Geometry: see drawing. Coordinates: mm, zero at the bounding-box minimum. Give positions to 0.01 mm unless a question says otherwise; leave off trailing zeros. Order: outer loops, then holes, each group sorted by start corner. A loop starts at its lowest first (then second) coordinate and runs counter-clockwise, first axis right, second up. Notation, with made-up numbers: (43, 20) - (82, 20) arc R10 cw to (82, 29) - close; hole circle Ø8 at (-12.75, 58). An arc over 180 degrees is marked (long way). One line per question, with ' | ' between items. Start each with the question number.
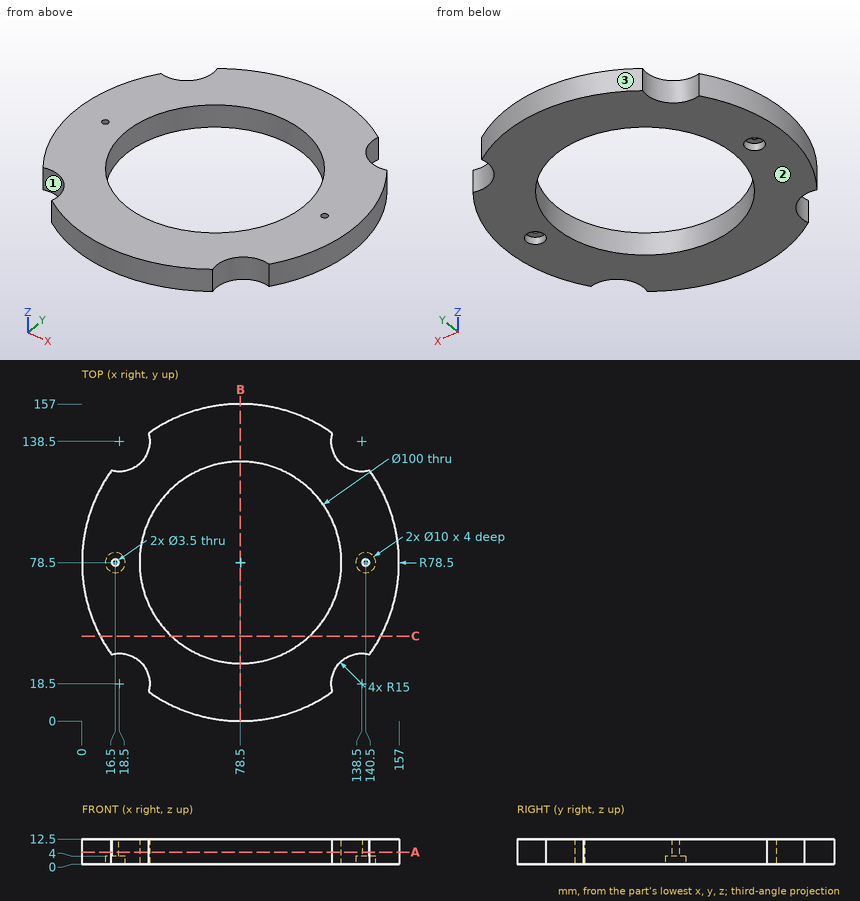
(1) Cut plane A-A, the plane z = 6. Return the cut outline in (x, y), plus the area to 3 significant figures.
(2) Pull-direction query (X, two-part tool) for the marked faces 1, 2 and 3; classes: +X half, -X half, draft (parallel to the pull), parting line (faces both ways), or undercut.
(3) Cut plane B-B, the plane x = 78.5. Return the cut outline in (y, z).
(4) Contact query for flat-ended pins moving along their axis: P1, Ø8, axis at x = 141, y = 78.5, coming from the -Z side; P2, Ø5, axis at y = 43.5, z = 5, coming from the +X side; P3, Ø2, axis at x = 16.5, y = 78.5, coming from the -Z side; P4, Ø1.5, axis at y = 22, z = 9.5, coming from the -X side. Output: stop coordinate, or through.
(5) Cut plane C-C, the plane y = 42. Return the cut outline in (x, z).
(6) Material intervals for line 1 along Y through (x, z) = (78.5, 9.25); line 2 along X through (y, z) = (106, 9.5); line 3 along Y through (x, z) = (113.5, 8.5), sorted ascending. Write a range as from..to.
Results are:
1) outline: (14.55, 32.97) arc R15 cw to (32.97, 14.55) arc R78.5 ccw to (124.03, 14.55) arc R15 cw to (142.45, 32.97) arc R78.5 ccw to (142.45, 124.03) arc R15 cw to (124.03, 142.45) arc R78.5 ccw to (32.97, 142.45) arc R15 cw to (14.55, 124.03) arc R78.5 ccw to start; hole circle Ø3.5 at (16.5, 78.5); hole circle Ø100 at (78.5, 78.5); hole circle Ø3.5 at (140.5, 78.5) | area: 10,900 mm2
2) face 1: undercut | face 2: draft | face 3: parting line
3) outline: (0, 0) - (28.5, 0) - (28.5, 12.5) - (0, 12.5) - close; (128.5, 0) - (157, 0) - (157, 12.5) - (128.5, 12.5) - close
4) P1: z = 4 | P2: x = 149.96 | P3: through | P4: x = 32.89
5) outline: (9, 0) - (44.33, 0) - (44.33, 12.5) - (9, 12.5) - close; (112.67, 0) - (148, 0) - (148, 12.5) - (112.67, 12.5) - close
6) line 1: 0..28.5, 128.5..157 | line 2: 4.97..36.74, 120.26..152.03 | line 3: 8.23..42.79, 114.21..148.77
